Check sheet for the modelled part. Datum: model origin and axes. Units: mm. Face numbers are marked on the shaded views. A direction names the side the tool comes from. Coordinates: 2 decimals unless noted, no trailing zeros. Write each loop counter-clockwise with the first axis right and the second up, starting at its lowest first coordinate (ties: lowest second). Pieces come first, ordered by that corner, then holes. Notation, with made-up numbers: (56.25, 11.25) - (67.25, 11.25) arc R19 ccw to (67.25, 26.25) - close; hole circle Ø6 at (12, 35.5). An arc over 180 degrees is marked (long way). Answer as CSV lines item,"result". Start each with the question number.
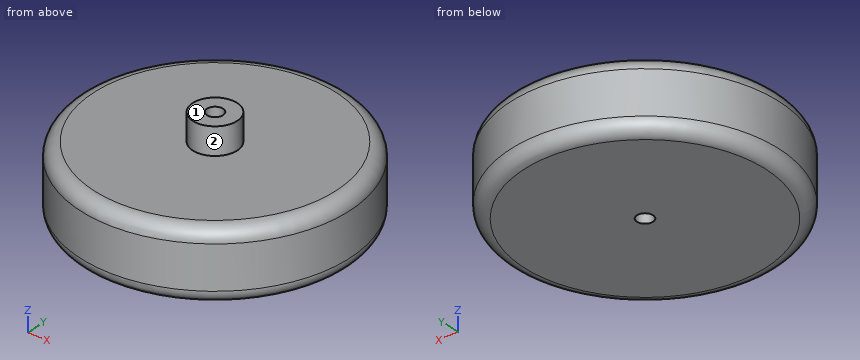
from build123d import *

# Parameters (mm, degrees)
SKETCH1_R           = 50
SKETCH1_R_2         = 3
BOSS_EXTRUDE1_DEPTH = 26
FILLET2_R           = 5
SKETCH3_R           = 8.248611849
BOSS_EXTRUDE2_DEPTH = 10
CUT_EXTRUDE1_START  = -26
SKETCH4_R           = 3
CUT_EXTRUDE1_DEPTH  = 26


with BuildPart() as part:
    # Sketch1 → Boss-Extrude1 (new body)
    with BuildSketch(Plane.XY):
        with Locations(Location((0, 0, 0), (0, 0, 180))):
            Circle(SKETCH1_R)
        with Locations(Location((0, 0, 0), (0, 0, 180))):
            Circle(SKETCH1_R_2, mode=Mode.SUBTRACT)
    extrude(amount=BOSS_EXTRUDE1_DEPTH)

    # Fillet2
    fillet2_edges = [part.edges().sort_by_distance(p)[0] for p in [
        (50, 0, 0),
        (50, 0, 26),
    ]]
    fillet(fillet2_edges, radius=FILLET2_R)

    # Sketch3 → Boss-Extrude2 (add)
    with BuildSketch(Plane.XY.offset(26)):
        Circle(SKETCH3_R)
    extrude(amount=BOSS_EXTRUDE2_DEPTH)

    # Sketch4 → Cut-Extrude1 (cut)
    with BuildSketch(Plane.XY.offset(36).offset(CUT_EXTRUDE1_START)):
        with Locations(Location((0, 0, 0), (0, 0, 180))):
            Circle(SKETCH4_R)
    extrude(amount=CUT_EXTRUDE1_DEPTH, mode=Mode.SUBTRACT)


solid = part.part
(1) Cross-section at C-C on z = 7. Record the boundary of the cut face in (x, y).
(2) Tool access check on the marked faces 1 and 2. Record the directions out of +Z, -Z, +X, -X, +Y, -Y that give a thin tool (end or side, any length) a straight path to the whole face; none if there is none.
(3) Material ranges on probe 1 along Y at (x, z) = (0, 21); probe 2 along Z at (x, y) = (-44, -11); probe 3 along Y at (x, z) = (0, 24), recorded low to high. Write a range as from..to.
(4) Cross-section at A-A on y = 0. Record the boundary of the cut face in (x, z).
(5) Cross-section at D-D on z = 27.5. Record the boundary of the cut face in (x, y), plus the area to 3 significant figures.
(6) Go/stop test with flat-tipped pins: P1, Ø10, axis at y = -29, z = 17, coming from the -X side; P2, Ø8, axis at y = -32.5, z = 20.5, coming from the +X side; P3, Ø12, axis at y = 17, z = 31.5, coming from the -X side. Record where each tip stops, or that it passes through.
Checked values:
1,outline,"circle Ø100 at (0, 0); hole circle Ø6 at (0, 0)"
2,face 1,"+Z, +X, -X, +Y, -Y"
2,face 2,"+Z"
3,probe 1,"-50..-3, 3..50"
3,probe 2,"0.01..25.99"
3,probe 3,"-49..-3, 3..49"
4,outline,"(-50, 5) arc R5 ccw to (-45, 0) - (-3, 0) - (-3, 36) - (-8.25, 36) - (-8.25, 26) - (-45, 26) arc R5 ccw to (-50, 21) - close; (3, 0) - (45, 0) arc R5 ccw to (50, 5) - (50, 21) arc R5 ccw to (45, 26) - (8.25, 26) - (8.25, 36) - (3, 36) - close"
5,outline,"circle Ø16.5 at (0, 0); hole circle Ø6 at (0, 0)"
5,area,"185 mm^2"
6,P1,"x = -43.86"
6,P2,"x = 41.08"
6,P3,"x = -44.19"
